Verification items for the finished model (mm, model axes). Face numbers are marked on the shaded views. A direction names the side the tool comes from. Round coordinates to 2 decimals unless told otherwise and drop trailing zeros. Order: outer loops, then holes, each group sorted by start corner. A loop starts at its lowest first (then second) coordinate and runs counter-clockwise, first axis right, second up. Notation, with made-up numbers: M 42.5,85.25 L 67.5,85.25 A16 ccw 67.5,94.25 Z; hole C -40,35.5 d7. An arc over 180 degrees is marked long. Use one line per item in the form item = value. Start each with the question number.
Item 1: Cross-section at A-A on x = -12. Enter the section's corners in (y, z), then the cut area to 3 significant figures.
Item 2: Cross-section at D-D on y = 1.5. Enter the section's corners in (x, z), then the cut area to 3 significant figures.
Item 3: Thickness scan on probe 1 along Y at (x, z) = (12, 14.05); probe 2 along Z at (x, y) = (-13, 12.25); probe 3 along X at (y, z) = (3.25, 9.75). Record the ranges inside material, lowest first. Write a range as [from, to].
Item 4: Go/stop test with flat-tipped pins: pin 1 Ø3.5 at (y, z) = (11, 6) entering from -X; pin 2 Ø8 at (x, y) = (14, 8.5) entering from -Z; pin 3 Ø1.5 at (y, z) = (11.5, 2.5) entering from +X; pin 4 Ø6.5 at (x, y) = (12, 7.5) entering from +Z. Record where each tip stops, or that it passes through.
Item 5: Release check for a two-part mould opening along Y. For the marked faces 4, 5, 6 and 7 record: +Y half, -Y half, draft (parallel to the pull), parting line (faces both ways), or undercut.
Item 6: Tool access check on the marked faces 1, 2 and 3. Record the directions out of +Z, -Z, +X, -X, +Y, -Y that give a thin tool (end or side, any length) a straight path to the whole face; none if there is none.
Item 7: Cross-section at C-C on z = 12. Enter the section's corners in (x, y).
Item 8: Cross-section at B-B on y = 7.5. Enter the section's corners in (x, z).
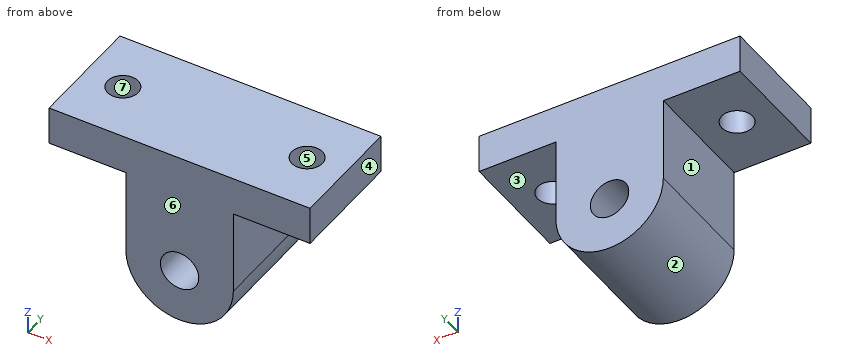
from build123d import *

# Parameters (mm, degrees)
ESQUISSE1_R             = 2.5
BOSS_EXTRU_1_DEPTH      = 15
ESQUISSE2_R             = 2
ENL_V_MAT_EXTRU_1_DEPTH = 15


with BuildPart() as part:
    # Esquisse1 → Boss.-Extru.1 (new body)
    with BuildSketch(Plane(origin=(0, 0, 0), x_dir=(1, 0, 0), z_dir=(0, 1, 0))):
        with BuildLine():
            Line((-7, 0), (-7, -11))
            Line((-7, -11), (-17, -11))
            Line((-17, -11), (-17, -16))
            Line((-17, -16), (17, -16))
            Line((17, -16), (17, -11))
            Line((17, -11), (7, -11))
            Line((7, -11), (7, 0))
            ThreePointArc((7, 0), (0, 7), (-7, 0))
        make_face()
        with Locations(Location((0, 0, 0), (0, 0, 270))):
            Circle(ESQUISSE1_R, mode=Mode.SUBTRACT)
    extrude(amount=BOSS_EXTRU_1_DEPTH)

    # Esquisse2 → Enlèv. mat.-Extru.1 (cut)
    with BuildSketch(Plane(origin=(0, 0, 11), x_dir=(-1, 0, 0), z_dir=(0, 0, -1))):
        with Locations((12, 7.5)):
            Circle(ESQUISSE2_R)
    enl_v_mat_extru_1 = extrude(amount=-ENL_V_MAT_EXTRU_1_DEPTH, mode=Mode.SUBTRACT)

    # Symétrie1: Enlèv. mat.-Extru.1 across plane
    add(enl_v_mat_extru_1.mirror(Plane(origin=(0, 0, 0), x_dir=(0, 0, 1), z_dir=(1, 0, 0))), mode=Mode.SUBTRACT)


solid = part.part
Output values:
q1.outline = M 0,11 L 5.5,11 L 5.5,16 L 0,16 Z; M 9.5,11 L 15,11 L 15,16 L 9.5,16 Z
q1.area = 55.0 mm2
q2.outline = M -17,11 L -7,11 L -7,0 A7 ccw 7,0 L 7,11 L 17,11 L 17,16 L -17,16 Z; hole C 0,0 d5
q2.area = 381 mm2
q3.probe_1 = [0, 5.5], [9.5, 15]
q3.probe_2 = [11, 16]
q3.probe_3 = [-7, 7]
q4.pin_1 = -7
q4.pin_2 = 11
q4.pin_3 = 7
q4.pin_4 = 16
q5.face_4 = draft
q5.face_5 = undercut
q5.face_6 = -Y half
q5.face_7 = undercut
q6.face_1 = -Z, -X, +Y, -Y
q6.face_2 = -Z, +Y, -Y
q6.face_3 = -Z, +X, +Y, -Y
q7.outline = M -17,0 L 17,0 L 17,15 L -17,15 Z; hole C -12,7.5 d4; hole C 12,7.5 d4
q8.outline = M -17,11 L -14,11 L -14,16 L -17,16 Z; M -10,11 L -7,11 L -7,0 A7 ccw 7,0 L 7,11 L 10,11 L 10,16 L -10,16 Z; M 14,11 L 17,11 L 17,16 L 14,16 Z; hole C 0,0 d5
